from build123d import *

# Parameters (mm, degrees)
F0_W      = 19.8
F0_H      = 55
F1_DEPTH  = 4.8
F2_R      = 5.75
F3_DEPTH  = 4.8
F4_R      = 6.3
F5_DEPTH  = 3.5
F6_W      = 4.8
F6_H      = 5
F7_DEPTH  = 5
F8_SIZE   = 4.99999
F9_W      = 4.8
F9_H      = 5
F10_DEPTH = 5
F11_SIZE  = 4.99999
F12_R     = 5
F13_DEPTH = 0.1
F14_DEPTH = 0.1


# Not quite as in the source:
# - a fillet or chamfer is up to 0.001 mm smaller than in the source, because OpenCascade refuses the exact size


with BuildPart() as f1:
    # F0 (on Front) → F1 (new body)
    with BuildSketch(Plane.XZ):
        with Locations((-0.9316042997, 16.8101646874)):
            Rectangle(F0_W, F0_H)
    extrude(amount=F1_DEPTH)

    # F2 (on face) → F3 (cut, through all)
    with BuildSketch(Plane.XZ.offset(4.8)):
        with Locations((-0.9316042997, 36.3101646874)):
            Circle(F2_R)
    extrude(amount=-F3_DEPTH, mode=Mode.SUBTRACT)

    # F4 (on face) → F5 (cut)
    with BuildSketch(Plane.XZ.offset(4.8)):
        with Locations((-0.9316042997, 36.3101646874)):
            Circle(F4_R)
    extrude(amount=-F5_DEPTH, mode=Mode.SUBTRACT)

    # F6 (on face) → F7 (join)
    with BuildSketch(Plane(origin=(-10.8316042997, 0, 0), x_dir=(0, -1, 0), z_dir=(-1, 0, 0))):
        with Locations((2.4, -3.1898353126)):
            Rectangle(F6_W, F6_H)
    extrude(amount=F7_DEPTH)

    # F8 (size 5 in the source; OpenCascade refuses exactly that, so slightly less here)
    f8_edges = [f1.edges().sort_by_distance(p)[0] for p in [
        (-15.831604, -2.4, -0.689835),
    ]]
    chamfer(f8_edges, length=F8_SIZE)

    # F9 (on face) → F10 (join)
    with BuildSketch(Plane.YZ.offset(8.9683957003)):
        with Locations((-2.4, -3.1898353126)):
            Rectangle(F9_W, F9_H)
    extrude(amount=F10_DEPTH)

    # F11 (size 5 in the source; OpenCascade refuses exactly that, so slightly less here)
    f11_edges = [f1.edges().sort_by_distance(p)[0] for p in [
        (13.968396, -2.4, -0.689835),
    ]]
    chamfer(f11_edges, length=F11_SIZE)

    # F12
    f12_edges = [f1.edges().sort_by_distance(p)[0] for p in [
        (-10.831604, -2.4, 44.310165),
        (8.968396, -2.4, 44.310165),
    ]]
    fillet(f12_edges, radius=F12_R)

    # F13 (cut): a face of the model
    f13_faces = [f1.faces().sort_by_distance(p)[0] for p in [
        (-10.8316042997, -2.4, -8.1898353126),
    ]]
    extrude(f13_faces, amount=-F13_DEPTH, mode=Mode.SUBTRACT)

    # F14 (cut): a face of the model
    f14_faces = [f1.faces().sort_by_distance(p)[0] for p in [
        (8.9683957003, -2.4, -8.1898353126),
    ]]
    extrude(f14_faces, amount=-F14_DEPTH, mode=Mode.SUBTRACT)


solid = f1.part
Can you work these out from the model? Positions are in its coordinate system, mm. A direction names the side the tool comes from. Give positions to 0.01 mm unless a question says otherwise; leave off trailing zeros. Loops run counter-clockwise (first coordinate to the right, second up) from the corner with the lowest first, then second, coordinate; pieces in that order, holes last. Notation, with made-up numbers: M 40.25,85 L 86.25,85 A23 cw 86.25,111 Z; hole C 6,82.25 d6. An arc over 180 degrees is marked long. One line per item, written item: value. Start each with the question number.
1) If we section it at A-A, the plane x = 2.5: Write out the boundary of the cut face in (y, z).
2) On a 3-axis mill with a long thin cutter (end or side, diameter ignored), from which of +Z, -Z, +X, -X, +Y, -Y can I reach the whole of each face in a straight line? I mean faces 1 (the face through (-10.832, -2, 19)), 2 (the face through (8.868, -2, -8)), 3 (the face through (-1, -2, 44.31)), 4 (the face through (-10.732, -2, -8)). Say none if no direction works.
3) Thinking about a two-plate mould opening in X: for faces 5 (the face through (-5.931, -3.074, 32.477)), 6 (the face through (8.968, -2, 19)), 7 (the face through (-13.297, -2.366, -3.155)), 8 (the face through (2, -1.3, 31)), which applies, +X half, -X half, draft (parallel to the pull), parting line (faces both ways), or undercut?
4) If we section it at C-C, the plane z = 32: Write out the boundary of the cut face in (x, y).
5) I'm going to push flat-ended pins straight in: pin 1 (2.5 mm diameter, centred on y = -3, z = -7, fed in from -X); pin 2 (2.5 mm diameter, centred on y = -3.5, z = 18, fed in from -X); pin 3 (2.5 mm diameter, centred on y = -2, z = -9.5, fed in from +X). Where does each tip first touch, or does it pass through?
6) If I drill on line 1 (X direction, y = -1.85, z = 19); line 2 (X direction, y = -1, z = -6.5); line 3 (X direction, y = -1.1, z = 31), over which ranges is the centre line in solid material (lowest first)? Write a range as [from, to].
7) If we section it at D-D, the plane z = 10: Write out the boundary of the cut face in (x, y), and give its area (3 significant figures).
Completed:
1. outline: M -4.8,-10.69 L 0,-10.69 L 0,31.7 L -1.3,31.7 L -1.3,31.03 L -4.8,31.03 Z; M -4.8,41.59 L -1.3,41.59 L -1.3,40.92 L 0,40.92 L 0,44.31 L -4.8,44.31 Z
2. face 1: +Z, -X, +Y, -Y
2. face 2: -Z, +X, +Y, -Y
2. face 3: +Z, +X, -X, +Y, -Y
2. face 4: -Z, -X, +Y, -Y
3. face 5: undercut
3. face 6: +X half
3. face 7: -X half
3. face 8: undercut
4. outline: M -10.83,-4.8 L -5.53,-4.8 L -5.53,-1.3 L -4.74,-1.3 L -4.74,0 L -10.83,0 Z; M 2.87,-1.3 L 3.66,-1.3 L 3.66,-4.8 L 8.97,-4.8 L 8.97,0 L 2.87,0 Z
5. pin 1: stops at x = -10.73
5. pin 2: stops at x = -10.83
5. pin 3: stops at x = 8.87
6. line 1: x = [-10.83, 8.97]
6. line 2: x = [-10.73, 8.87]
6. line 3: x = [-10.83, -3.14], [1.27, 8.97]
7. outline: M -10.83,-4.8 L 8.97,-4.8 L 8.97,0 L -10.83,0 Z
7. area: 95.0 mm^2
